Part model, mm, in its own coordinate system. Coordinates: 2 decimals unless noted, no trailing zeros. Loops run counter-clockwise (first coordinate to the right, second up) from the corner with the lowest first, then second, coordinate; pieces in that order, holes last. Notation, with made-up numbers: (39.25, -28.75) - (82.25, -28.75) arc R25 cw to (82.25, 8.25) - close; hole circle Ø1 at (67, 45.25). An arc over 180 degrees is marked (long way). Use a Markdown table: item, result. Add a question column.
1) Band-saw the part on A-A (z = 0). Give the cut face in (x, y) (3 decimals).
2) Probe probe 1 along X at (y, z) = (1.8, 13); probe 2 along Z at (x, y) = (20, 1.45) (3 decimals); probe 3 along Z at (x, y) = (-17, 0.75) (3 decimals). List the from-to ranges inside material, lowest first. Write a range as [from, to].
3) Band-saw the part on B-B (x = 0). Give the cut face in (y, z) (3 decimals), plus the area to 3 significant figures.
4) Pull direction Z, two halves, no side cores. Call faces 1 (the face through (0, 2, -15.875)), 2 (the face through (0.354, 1.565, 12.706)), 3 (the face through (0, 3.175, 0)): +Z half, -Z half, draft (parallel to the pull), parting line (faces both ways), or undercut.
5) Band-saw the part on C-C (y = 1.65). Give the number of separate pieces and of enclosed holes in the cut face, plus the area to 3 significant figures.
6) Drop a flat-ended pin along its axis: P1, Ø2, axis at x = 0, z = -11.11, coming from the -Y side. Give the stop position or say it passes through.
from build123d import *

# Parameters (mm, degrees)
SKETCH1_W              = 46.0375
SKETCH1_H              = 31.75
BOSS_EXTRUDE1_DEPTH    = 3.175
F_10_CLEARANCE_HOLE1_D = 5.1054
F_4_CLEARANCE_HOLE1_D  = 3.2639


with BuildPart() as part:
    # Sketch1 → Boss-Extrude1 (new body)
    with BuildSketch(Plane(origin=(0, 0, 0), x_dir=(1, 0, 0), z_dir=(0, 1, 0))):
        Rectangle(SKETCH1_W, SKETCH1_H)
    extrude(amount=BOSS_EXTRUDE1_DEPTH)

    # #10 Clearance Hole1 (through all)
    with Locations(Plane(origin=(0, 3.175, 0), x_dir=(1, 0, 0), z_dir=(0, 1, 0))):
        with Locations((-18.25625, 11.1125), (-18.25625, -11.1125), (18.25625, -11.1125), (18.25625, 11.1125)):
            Hole(F_10_CLEARANCE_HOLE1_D / 2)

    # #4 Clearance Hole1 (through all)
    with Locations(Plane(origin=(0, 3.175, 0), x_dir=(1, 0, 0), z_dir=(0, 1, 0))):
        with Locations((0, 11.1125), (0, -11.1125), (-18.25625, 0), (18.25625, 0)):
            Hole(F_4_CLEARANCE_HOLE1_D / 2)


solid = part.part
Answer block:
| question | item | result |
|---|---|---|
| 1 | outline | (-23.019, 0) - (-19.888, 0) - (-19.888, 3.175) - (-23.019, 3.175) - close; (-16.624, 0) - (16.624, 0) - (16.624, 3.175) - (-16.624, 3.175) - close; (19.888, 0) - (23.019, 0) - (23.019, 3.175) - (19.888, 3.175) - close |
| 2 | probe 1 | [-23.02, -19.97], [-16.54, 16.54], [19.97, 23.02] |
| 2 | probe 2 | [-15.875, -12.977], [-9.248, 9.248], [12.977, 15.875] |
| 2 | probe 3 | [-15.875, -13.335], [-8.89, -1.042], [1.042, 8.89], [13.335, 15.875] |
| 3 | outline | (0, -15.875) - (3.175, -15.875) - (3.175, -12.744) - (0, -12.744) - close; (0, -9.481) - (3.175, -9.481) - (3.175, 9.481) - (0, 9.481) - close; (0, 12.744) - (3.175, 12.744) - (3.175, 15.875) - (0, 15.875) - close |
| 3 | area | 80.1 mm2 |
| 4 | face 1 | -Z half |
| 4 | face 2 | undercut |
| 4 | face 3 | draft |
| 5 | separate pieces | 1 |
| 5 | enclosed holes | 8 |
| 5 | area | 1,350 mm2 |
| 6 | P1 | through |
